from build123d import *

# Parameters (mm, degrees)
SKETCH1_R           = 20
BOSS_EXTRUDE1_DEPTH = 10
SKETCH2_R           = 4
CUT_EXTRUDE1_DEPTH  = 11
SKETCH3_R           = 12.5
CUT_EXTRUDE2_DEPTH  = 2
FILLET1_R           = 2


with BuildPart() as part:
    # Sketch1 → Boss-Extrude1 (new body)
    with BuildSketch(Plane.XY):
        Circle(SKETCH1_R)
    extrude(amount=BOSS_EXTRUDE1_DEPTH)

    # Sketch2 → Cut-Extrude1 (cut, through all)
    with BuildSketch(Plane.XY):
        Circle(SKETCH2_R)
    extrude(amount=CUT_EXTRUDE1_DEPTH, mode=Mode.SUBTRACT)

    # Sketch3 → Cut-Extrude2 (cut)
    with BuildSketch(Plane.XY.offset(10)):
        Circle(SKETCH3_R)
    extrude(amount=-CUT_EXTRUDE2_DEPTH, mode=Mode.SUBTRACT)

    # Fillet1
    fillet1_edges = [part.edges().sort_by_distance(p)[0] for p in [
        (-20, 0, 0),
        (-20, 0, 10),
    ]]
    fillet(fillet1_edges, radius=FILLET1_R)


solid = part.part
Input: part model. Units: mm. Frame: model coordinates. A direction names the side the tool comes from. Coordinates: 2 decimals unless noted, no trailing zeros. Loops run counter-clockwise (first coordinate to the right, second up) from the corner with the lowest first, then second, coordinate; pieces in that order, holes last.
Q1. Set-up query: faces 1 (the face through (11.923, 3.755, 9.014)), 2 (the face through (-4.3, 0.3, 0)). Return all of +Z, -Z, +X, -X, +Y, -Y with unobstructed straight access to the full face (end or side cutting, diameter ignored); none if empty.
Q2. Cut plane A-A (y = 0). Output: boundary loops of the cut face in (x, z), then the cut area to 3 significant figures.
Q3. Cut plane C-C (z = 3). Output: boundary loops of the cut face in (x, y).
Q4. Material intervals for line 1 (Y direction, x = 0, z = 6); line 2 (X direction, y = -0.5, z = 8.5); line 3 (Z direction, x = 0.5, y = 5.5), sorted ascending.
Q5. Contact query for flat-ended pins moving along their axis: pin 1 (1.5 mm diameter, centred on y = 11.5, z = 8, fed in from -X); pin 2 (3 mm diameter, centred on y = -11, z = 8, fed in from +X); pin 3 (1 mm diameter, centred on y = -6.5, z = 4, fed in from +X). Output: stop coordinate, or through.
Q6. Draft query along Y for faces 3 (the face through (-0.867, -3.905, 3.944)), 4 (the face through (-12.3, -3.7, 10)), 5 (the face through (-4.336, -19.524, 4.958)), 6 (the face through (-3, 3, 8)). Return one class per face: +Y half, -Y half, draft (parallel to the pull), parting line (faces both ways), or undercut.
Working result:
1. face 1: +Z
1. face 2: -Z, +X, -X, +Y, -Y
2. outline: (-20, 2) arc R2 ccw to (-18, 0) - (-4, 0) - (-4, 8) - (-12.5, 8) - (-12.5, 10) - (-18, 10) arc R2 ccw to (-20, 8) - close; (4, 0) - (18, 0) arc R2 ccw to (20, 2) - (20, 8) arc R2 ccw to (18, 10) - (12.5, 10) - (12.5, 8) - (4, 8) - close
2. area: 283 mm2
3. outline: circle Ø40 at (0, 0); hole circle Ø8 at (0, 0)
4. line 1: y = -20 to -4, 4 to 20
4. line 2: x = -19.93 to -12.49, 12.49 to 19.93
4. line 3: z = 0 to 8
5. pin 1: stops at x = -16.87
5. pin 2: stops at x = 17.6
5. pin 3: stops at x = 19.08
6. face 3: undercut
6. face 4: draft
6. face 5: parting line
6. face 6: undercut
